Build history of the part. All positions in model axes, mm. Face numbers are marked on the shaded views. A direction names the side the tool comes from. Give positions to 0.01 mm unless a question says otherwise; leave off trailing zeros. Loops run counter-clockwise (first coordinate to the right, second up) from the corner with the lowest first, then second, coordinate; pieces in that order, holes last. Notation, with made-up numbers: M 38.5,0.5 L 74.5,0.5 A30 cw 74.5,23.5 Z; hole C -4.75,2.25 d1. An arc over 180 degrees is marked long. Answer in a Markdown table with one row per item. Add a question column.
```python
from build123d import *

# Parameters (mm, degrees)
F0_W     = 40
F0_H     = 5
F1_DEPTH = 90
F2_W     = 7
F2_H     = 30.4702166427
F2_H_2   = 30
F3_DEPTH = 240
F5_D     = 9


# Not quite as in the source:
# - a feature names something its author has since deleted; it is built from what else it names


with BuildPart() as f1:
    # F0 (on Right) → F1 (new body)
    with BuildSketch(Plane.YZ):
        with Locations((-0.72813743, 2.5)):
            Rectangle(F0_W, F0_H)
    extrude(amount=F1_DEPTH)

    # F2 (on Top) → F3 (join)
    with BuildSketch(Plane.XY):
        with Locations((31, -0.7447636027)):
            Rectangle(F2_W, F2_H)
        with Locations((59, -0.72813743)):
            Rectangle(F2_W, F2_H_2)
    extrude(amount=F3_DEPTH)

    # F5 (through all)
    with Locations(Plane(origin=(0, 0, 0), x_dir=(1, 0, 0), z_dir=(0, 0, -1))):
        with Locations((13, 0), (77, 0)):
            Hole(F5_D / 2)


solid = f1.part
```
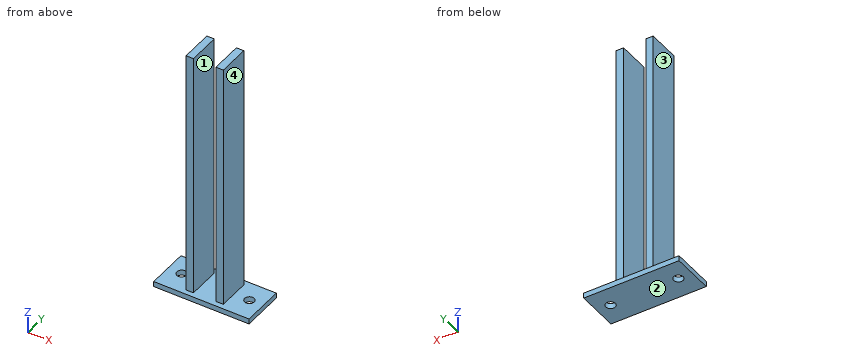
(1) Slice it at B-B, the plane y = 0. Give the cut face in (x, z), then the cut area to 3 significant figures.
(2) Slice it at A-A, the plane x = 13. Give the cut face in (y, z).
(3) Slice it at D-D, the plane y = 10.5. Give the cut face in (x, z).
(4) Wall check: line 1 (X direction, y = -13, z = 206); line 2 (Y direction, x = 13, z = 2.1); line 3 (Z direction, x = 61, y = 17.5). Give the ranges that are in metal, low to high.
(5) Tool access for the marked faces 1, 2, 3 and 4: list every direction of +Z, -Z, +X, -X, +Y, -Y with a clear straight run to the whole face (end or side of a thin tool).
(6) Pin check, flat tips, straight feed: pin 1 (5.5 mm diameter, centred on x = 30.5, z = 148.5, fed in from +Y); pin 2 (9 mm diameter, centred on y = 3.5, z = 151.5, fed in from +X); pin 3 (6 mm diameter, centred on x = 74, y = -9, fed in from +Z). Stop position of each tip, or through.
(7) Slice it at C-C, the plane z = 94. Give the cut face in (x, y), then the cut area to 3 significant figures.
Solution:
| question | item | result |
|---|---|---|
| 1 | outline | M 0,0 L 8.5,0 L 8.5,5 L 0,5 Z; M 17.5,0 L 72.5,0 L 72.5,5 L 62.5,5 L 62.5,240 L 55.5,240 L 55.5,5 L 34.5,5 L 34.5,240 L 27.5,240 L 27.5,5 L 17.5,5 Z; M 81.5,0 L 90,0 L 90,5 L 81.5,5 Z |
| 1 | area | 3,650 mm^2 |
| 2 | outline | M -20.73,0 L -4.5,0 L -4.5,5 L -20.73,5 Z; M 4.5,0 L 19.27,0 L 19.27,5 L 4.5,5 Z |
| 3 | outline | M 0,0 L 90,0 L 90,5 L 62.5,5 L 62.5,240 L 55.5,240 L 55.5,5 L 34.5,5 L 34.5,240 L 27.5,240 L 27.5,5 L 0,5 Z |
| 4 | line 1 | 27.5 to 34.5, 55.5 to 62.5 |
| 4 | line 2 | -20.73 to -4.5, 4.5 to 19.27 |
| 4 | line 3 | 0 to 5 |
| 5 | face 1 | +Z, +Y, -Y |
| 5 | face 2 | -Z, +X, -X, +Y, -Y |
| 5 | face 3 | +Z, -X, +Y, -Y |
| 5 | face 4 | +Z, +X, +Y, -Y |
| 6 | pin 1 | y = 14.49 |
| 6 | pin 2 | x = 62.5 |
| 6 | pin 3 | z = 5 |
| 7 | outline | M 27.5,-15.98 L 34.5,-15.98 L 34.5,14.49 L 27.5,14.49 Z; M 55.5,-15.73 L 62.5,-15.73 L 62.5,14.27 L 55.5,14.27 Z |
| 7 | area | 423 mm^2 |
